Part print with two shaded views. Sizes in mm from the minimum x, y, z corner. A direction names the side the tool comes from. Round coordinates to 2 decimals unless told otherwise and drop trailing zeros. Loops run counter-clockwise (first coordinate to the right, second up) from the corner with the lowest first, then second, coordinate; pieces in that order, holes last. Notation, with made-up numbers: (43, -4) - (83, -4) arc R8 cw to (83, 4) - close; hole circle Ø4 at (44, -25.75). An arc over 180 degrees is marked (long way). Put each result on its own line as item: value. Start each with the question number.
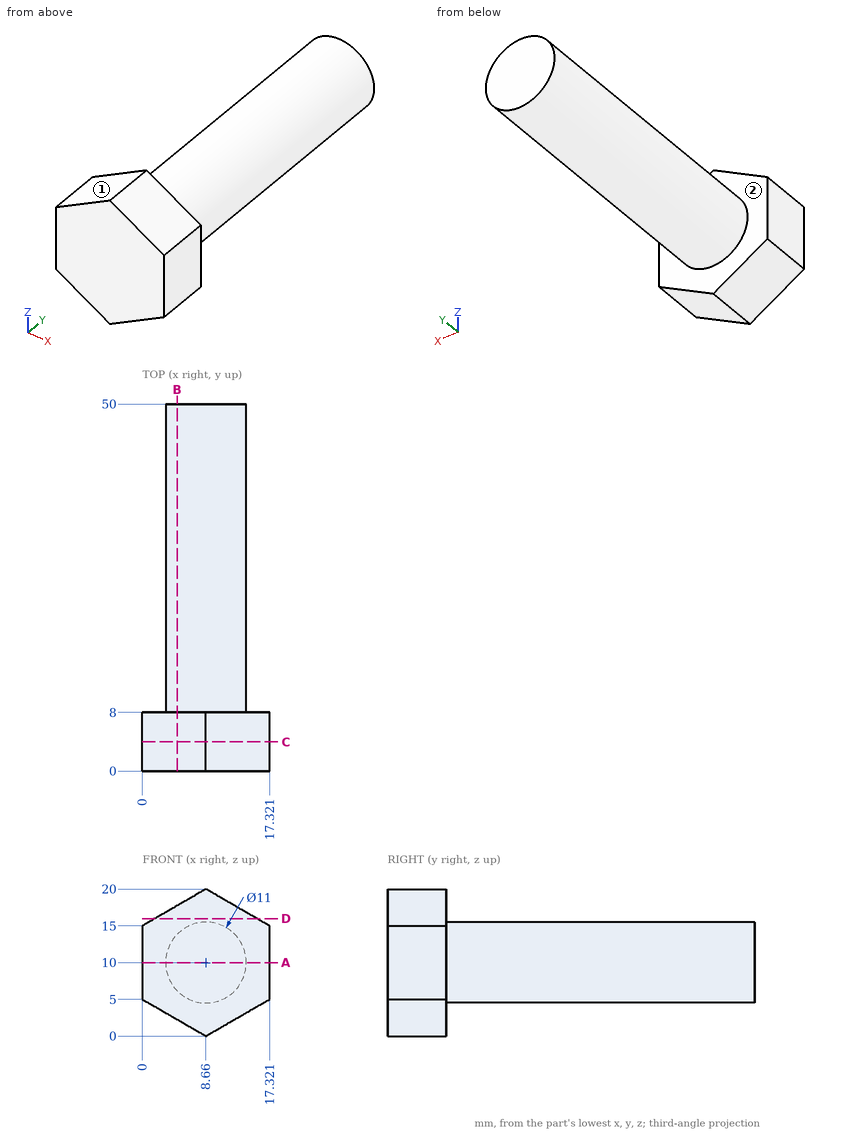
1) Slice it at D-D, the plane z = 16. Write the cut outline in (x, y), and give its area (3 significant figures).
2) Slice it at A-A, the plane z = 10. Write the cut outline in (x, y).
3) Slice it at C-C, the plane y = 4. Write the cut outline in (x, z).
4) Slice it at B-B, the plane x = 4.75. Write the cut outline in (y, z).
5) Which spindle directions (+Z, -Z, +X, -X, +Y, -Y) get a long thin tool onto all of the face, cutting with end or side? Do the marked faces 1 and 2. Say none if no direction does.
6) Drill centre lines: line 1 (Z direction, x = 9, y = 11); line 2 (Y direction, x = 14, z = 4.25); line 3 (X direction, y = 20, z = 5.75). Where is each one in solid material? Low to high. Write a range as [from, to].
7) Drop flat-ended pins along their axis: pin 1 Ø1 at (x, y) = (9, 36.5) entering from +Z; pin 2 Ø12 at (y, z) = (20, 7) entering from +X; pin 3 Ø6 at (y, z) = (42, 2.5) entering from +X (1 decimal). Give the stop position or say it passes through.
Taken from the geometry:
1. outline: (1.73, 0) - (15.59, 0) - (15.59, 8) - (1.73, 8) - close
1. area: 111 mm2
2. outline: (0, 0) - (17.32, 0) - (17.32, 8) - (14.16, 8) - (14.16, 50) - (3.16, 50) - (3.16, 8) - (0, 8) - close
3. outline: (0, 5) - (8.66, 0) - (17.32, 5) - (17.32, 15) - (8.66, 20) - (0, 15) - close
4. outline: (0, 2.26) - (8, 2.26) - (8, 6.13) - (50, 6.13) - (50, 13.87) - (8, 13.87) - (8, 17.74) - (0, 17.74) - close
5. face 1: +Z, -X, +Y, -Y
5. face 2: +Y
6. line 1: z = [4.51, 15.49]
6. line 2: y = [0, 8]
6. line 3: x = [5.17, 12.15]
7. pin 1: stops at z = 15.5
7. pin 2: stops at x = 14.16
7. pin 3: stops at x = 11.8
